Autodesk Inventor part; units mm, degrees
ref_plane "YZ Plane" through (0, 0, 0) normal (1, 0, 0) x (0, 1, 0)
ref_plane "XZ Plane" through (0, 0, 0) normal (0, 1, 0) x (-1, 0, 0)
ref_plane "XY Plane" through (0, 0, 0) normal (0, 0, 1) x (1, 0, 0)
sketch "Sketch1" plane through (0, 0, 0) normal (0, 0, 1) x (1, 0, 0)
  arc A0 (-85.6258, 79.4796) -> (-116.0775, 49.6172) centre (-86.1702, 49.5773) ccw
  line L0 (-85.6258, 79.4796) -> (33.3305, 79.4959)
  arc A1 (63.2389, 49.5916) -> (33.3305, 79.4959) centre (33.3346, 49.5916) ccw
  line L1 (63.2389, -50.9075) -> (63.2389, 49.5916)
  line L2 (63.2389, 49.5916) -> (63.2389, -53.5021)
  line L3 (-116.0775, 49.6172) -> (-116.3855, -51.7391)
  line L4 (-116.0775, 49.6172) -> (-116.0775, -50.4074)
  line L5 (-106.0129, -63.5021) -> (53.2389, -63.5021)
  arc A2 (53.2389, -63.5021) -> (63.2389, -53.5021) centre (53.2389, -53.5021) ccw
  arc A3 (-86.7039, 77.4795) -> (-114.0775, 49.6129) centre (-86.1702, 49.5773) ccw
  line L6 (-86.7039, 77.4795) -> (33.3308, 77.4959)
  arc A4 (61.2389, 49.5916) -> (33.3308, 77.4959) centre (33.3346, 49.5916) ccw
  line L7 (61.2389, 49.5916) -> (61.2389, -53.5021)
  arc A5 (53.2389, -61.5021) -> (61.2389, -53.5021) centre (53.2389, -53.5021) ccw
  line L8 (53.2389, -61.5021) -> (-106.0129, -61.5021)
  arc A6 (-114.3859, -51.8743) -> (-106.0129, -61.5021) centre (-106.0129, -53.0473) ccw
  line L9 (-114.3859, -51.8743) -> (-114.0775, 49.6129)
  line L10 (33.3308, 77.2959) -> (-85.6461, 77.2796)
  arc A7 (-85.6461, 77.2796) -> (-113.8775, 49.6124) centre (-86.1702, 49.5773) ccw
  line L11 (-113.8775, 49.6124) -> (-114.1859, -51.8886)
  arc A8 (-114.1859, -51.8886) -> (-106.0129, -61.3021) centre (-106.0129, -53.0473) ccw
  line L12 (-106.0129, -61.3021) -> (53.2389, -61.3021)
  arc A9 (53.2389, -61.3021) -> (61.0389, -53.5021) centre (53.2389, -53.5021) ccw
  line L13 (61.0389, -53.5021) -> (61.0389, 49.5916)
  arc A10 (61.0389, 49.5916) -> (33.3308, 77.2959) centre (33.3346, 49.5916) ccw
  circle A11 centre (-102.0292, 65.4774) radius 1.5
  circle A12 centre (49.2389, 65.498) radius 1.5
  circle A13 centre (-26.6496, -56.5021) radius 1.5
  circle A14 centre (-91.3999, -56.5021) radius 1.5
  circle A15 centre (38.2389, -56.5021) radius 1.5
  line L14 (-116.0775, -2.0021) -> (63.2389, -2.0021)
  line L15 (-43.7191, -2.0021) -> (-9.1191, -2.0021)
  line L16 (-9.1191, -2.0021) -> (-9.1191, -24.0021)
  line L17 (-9.1191, -24.0021) -> (-43.7191, -24.0021)
  line L18 (-43.7191, -24.0021) -> (-43.7191, -2.0021)
  circle A16 centre (-43.7191, -2.0021) radius 1.25
  circle A17 centre (-9.1191, -2.0021) radius 1.25
  circle A18 centre (-9.1191, -24.0021) radius 1.25
  circle A19 centre (-43.7191, -24.0021) radius 1.25
  line L19 (-63.7191, 9.7883) -> (-63.7191, -26.3021)
  circle A20 centre (-63.7191, 21.1979) radius 2
  circle A21 centre (-63.7191, -26.3021) radius 2
  line L20 (-63.7191, 21.1979) -> (-106.2191, 21.1979)
  line L21 (-63.7191, -26.3021) -> (-106.2191, -26.3021)
  line L22 (-106.2191, -26.3021) -> (-106.2191, 21.1979)
  circle A22 centre (-106.2191, 21.1979) radius 2
  circle A23 centre (-106.2191, -26.3021) radius 2
  line L23 (-63.7191, 9.7883) -> (-63.7191, 21.1979)
  line L24 (-109.1691, 24.1479) -> (-60.7691, 24.1479)
  line L25 (-60.7691, 24.1479) -> (-60.7691, 9.7883)
  line L26 (-60.7691, 9.7883) -> (-60.7691, -29.2521)
  line L27 (-60.7691, -29.2521) -> (-109.1691, -29.2521)
  line L28 (-109.1691, -29.2521) -> (-109.1691, 24.1479)
  line L29 (8.8809, 39.1979) -> (54.8809, 39.1979)
  line L30 (54.8809, 39.1979) -> (54.8809, -26.3021)
  line L31 (54.8809, -26.3021) -> (8.8809, -26.3021)
  line L32 (8.8809, -26.3021) -> (8.8809, 39.1979)
  circle A24 centre (8.8809, 39.1979) radius 2
  circle A25 centre (54.8809, 39.1979) radius 2
  circle A26 centre (8.8809, -26.3021) radius 2
  circle A27 centre (54.8809, -26.3021) radius 2
  circle A28 centre (-88.8693, 52.2792) radius 10
  point P0 (0, 0)
  point P1 (44.321, -53.9075)
  point P2 (51.321, -50.9075)
  point P3 (-9.1191, -13.0021)
  point P4 (-84.9691, -26.3021)
  dimension "d0" = 10
  dimension "d1" = 2
  dimension "d2" = 0.2
  dimension "d3" = 3
  dimension "d4" = 3
  dimension "d5" = 3
  dimension "d6" = 3
  dimension "d7" = 3
  dimension "d8" = 14
  dimension "d9" = 14
  dimension "d10" = 14
  dimension "d11" = 14
  dimension "d12" = 89.75
  dimension "d13" = 7
  dimension "d14" = 7
  dimension "d15" = 7
  dimension "d16" = 25
  dimension "d17" = 25
  dimension "d20" = 61.5
  dimension "d21" = 34.6
  dimension "d22" = 22
  dimension "d23" = 2.5
  dimension "d24" = 2.5
  dimension "d25" = 2.5
  dimension "d26" = 2.5
  dimension "d27" = 0
  dimension "d28" = 179.3164
  dimension "d29" = 72.358
  dimension "d32" = 20
  dimension "d33" = 47.5
  dimension "d34" = 4
  dimension "d35" = 4
  dimension "d36" = 42.5
  dimension "d37" = 4
  dimension "d38" = 4
  dimension "d39" = 48.4
  dimension "d51" = 46
  dimension "d52" = 65.5
  dimension "d53" = 18
  dimension "d54" = 35
  dimension "d55" = 35
  dimension "d56" = 4
  dimension "d57" = 4
  dimension "d58" = 4
  dimension "d59" = 4
  dimension "d62" = 20
  dimension "d63" = 25
  dimension "d64" = 25
  dimension "d67" = 27.7043
extrude "Extrusion1" add sketch "Sketch1" along normal blind 3 contours L14 L28 L27 L26 A16 L18 A19 L17 A18 L16 A17 L32 A26 L31 A27 L30 L13 A9 L12 A8 L11 | L11 A7 L10 A10 L13 L14 L30 A25 L29 A24 L32 A17 A16 L26 L25 L24 L28 | L28 L24 L25 L26 L14 L19 L23 A20 L20 A22 L22 | L14 L22 A23 L21 A21 L19 L26 L27 L28 | L22 A22 L20 A20 L23 L19 L14 | L14 L19 A21 L21 A23 L22 | L30 A27 L31 A26 L32 L14 | L14 L32 A24 L29 A25 L30 | A23 L21 L22 | L22 L21 A23 | A22 L20 L22 | L22 L20 A22 | A25 L29 L30 | L30 L29 A25 | A27 L31 L30 | L30 L31 A27 | A21 L21 L19 | L19 L21 A21 | A17 L16 L14 | L14 A17 | A26 L31 L32 | L32 L31 A26 | A24 L29 L32 | L32 L29 A24 | A16 L14 | L14 L18 A16 | L23 L20 A20 | A20 L20 L23 | L16 A17 L14 | A17 L16 A18 L17 A19 L18 A16 L14 | L14 A16 L18 | A18 L17 L16 | L16 L17 A18 | A19 L17 L18 | L18 L17 A19 | A28
extrude "Extrusion2" cut sketch "Sketch1" along normal up to surface (3 mm away) contours A17 L16 L14 | L14 A17 | A16 L14 | L14 L18 A16 | L16 A17 L14 | L14 A16 L18 | A18 L17 L16 | L16 L17 A18 | A19 L17 L18 | L18 L17 A19
extrude "Extrusion3" cut sketch "Sketch1" along normal blind 3 contours A23 L21 L22 | L22 L21 A23 | A22 L20 L22 | L22 L20 A22 | A21 L21 L19 | L19 L21 A21 | L23 L20 A20 | A20 L20 L23
extrude "Extrusion5" cut sketch "Sketch1" along normal up to surface (3 mm away) contours A25 L29 L30 | L30 L29 A25 | A27 L31 L30 | L30 L31 A27 | A26 L31 L32 | L32 L31 A26 | A24 L29 L32 | L32 L29 A24
extrude "Extrusion6" cut sketch "Sketch1" along normal blind 3 contours A28
properties part number "Final_Back_Cover_1"
Read the model definition and answer for the solid it produces. Units are mm, in the model's axes. Coordinates: 2 decimals unless noted, no trailing zeros. Write each loop counter-clockwise with the first axis right and the second up, starting at its lowest first coordinate (ties: lowest second). Pieces come first, ordered by that corner, then holes. Notation, with made-up numbers: (41.5, 18.25) -> (87.5, 18.25) arc R18 ccw to (87.5, 35.25) -> close; hole circle Ø11 at (-25, -17). An arc over 180 degrees is marked (long way). Return JSON: item names as keys, results as strings.
1. A cutting plane is placed at B-B (y = 47). Determine the outline of the cut face in (x, z), and give its area (3 significant figures).
Found:
{"outline": "(-113.89, 0) -> (-97.36, 0) -> (-97.36, 3) -> (-113.89, 3) -> close; (-80.38, 0) -> (61.04, 0) -> (61.04, 3) -> (-80.38, 3) -> close", "area": "474 mm2"}
2. Determine the mould class of faces 1 (the face through (-112.181, -58.533, 1.479)), 2 (the face through (-104.31, -26.9, 1.48)), 3 (the face through (9.956, 37.511, 1.479)), 4 (the face through (-28, 9, 3)) for opening direction X: pulls with the +X half, pulls with the -X half, needs draft (parallel to the pull), parting line crosses it, or undercut.
Found:
{"face 1": "pulls with the -X half", "face 2": "undercut", "face 3": "undercut", "face 4": "needs draft"}
3. Each of these flat-tipped pins is pushed along its axis until it touches: P1, Ø2.5, axis at x = -26.65, y = -56.5, coming from the +Z side; P2, Ø1.5, axis at x = -13, z = 1, coming from the +Y side. Where does it stop, or does it pass through?
Found:
{"P1": "through", "P2": "y = 77.29"}
4. A cutting plane is placed at A-A (z = 1.55). Give the number of separate pieces and of enclosed holes in the cut face, and give its area (3 significant figures).
Found:
{"separate pieces": "1", "enclosed holes": "18", "area": "23,400 mm2"}
5. Find the intervals of material crossed by line 1 along X through (y, z) = (66.5, 1.9); line 2 along X through (y, z) = (21.5, 1.35); line 3 along Y through (x, z) = (-32.5, 1.25), in increasing order. Write a range as from..to.
Found:
{"line 1": "-108.11..-103.13, -100.93..48.12, 50.36..55.28", "line 2": "-113.96..-108.2, -104.24..-65.7, -61.74..61.04", "line 3": "-61.3..77.29"}
